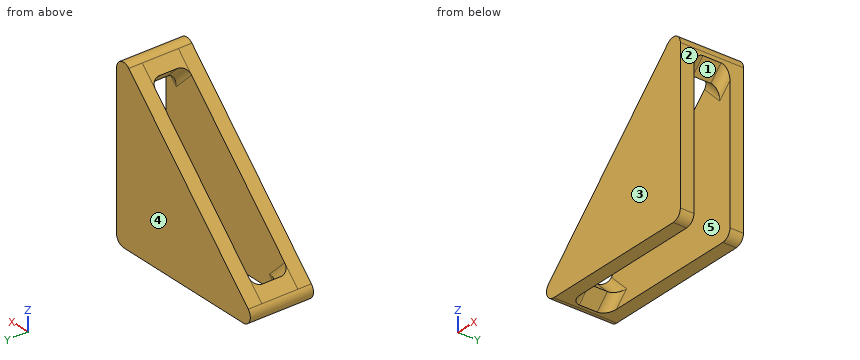
Autodesk Inventor part; units mm, degrees
ref_plane "YZ Plane" through (0, 0, 0) normal (1, 0, 0) x (0, 1, 0)
ref_plane "XZ Plane" through (0, 0, 0) normal (0, 1, 0) x (-1, 0, 0)
ref_plane "XY Plane" through (0, 0, 0) normal (0, 0, 1) x (1, 0, 0)
sketch "Sketch1" plane through (0, 0, 0) normal (0, 1, 0) x (-1, 0, 0)
  line L0 (0, 0) -> (-40, 0)
  line L1 (-40, 0) -> (-40, 40)
  line L2 (-40, 40) -> (0, 0)
  dimension "d0" = 40
  dimension "d1" = 40
  dimension "d2" = 56.5685
extrude "Extrusion1" add sketch "Sketch1" along normal blind 14
sketch "Sketch2" plane through (40, 0, 40) normal (-0.7071068, 0, 0.7071068) x (0.7071068, 0, 0.7071068)
  line L0 (-56.5685, 0) -> (-56.5685, 14) construction
  line L1 (-56.5685, 7) -> (0, 7) construction
  line L2 (0, 0) -> (0, 14) construction
  line L3 (-52.5685, 11) -> (-4, 11)
  line L4 (-4, 11) -> (-4, 3)
  line L5 (-4, 3) -> (-52.5685, 3)
  line L6 (-52.5685, 3) -> (-52.5685, 11)
  line L7 (-52.5685, 11) -> (-4, 3) construction
  line L8 (-4, 11) -> (-52.5685, 3) construction
  point P0 (-28.2843, 7)
  dimension "d5" = 4
  dimension "d6" = 4
  dimension "d20" = 8
extrude "Extrusion2" cut sketch "Sketch2" against normal blind 28.75
fillet "Fillet1" radius 2 4 edges at (40, 12.5, 0) (40, 1.5, 0) (40, 7, 40) (0, 7, 0)
sketch "Sketch4" plane through (5.6569, 3, 0) normal (0.7071068, 0, 0.7071068) x (0.7071068, 0, -0.7071068)
  line L0 (-3.8204, 0) -> (-3.8204, 8)
  line L1 (-3.8204, 0) -> (0, 0)
  line L2 (0, 8) -> (0, 0)
  line L3 (-3.8204, 8) -> (0, 8)
  point P0 (-4, -3)
extrude "Extrusion3" add sketch "Sketch4" along normal blind 4
sketch "Sketch5" plane through (40, 3, 34.3431) normal (-0.7071068, 0, -0.7071068) x (-0.7071068, 0, 0.7071068)
  line L0 (3.8204, 8) -> (3.8204, 0)
  line L1 (3.8204, 8) -> (0, 8)
  line L2 (0, 0) -> (0, 8)
  line L3 (3.8204, 0) -> (0, 0)
  point P0 (4, -3)
extrude "Extrusion4" add sketch "Sketch5" along normal blind 4
sketch "Sketch6" plane through (37.2986, 3, 37.0445) normal (-0.7071068, 0, 0.7071068) x (0.7071068, 0, 0.7071068)
  line L0 (0, 8) -> (0, 0)
  line L1 (-4, 8) -> (0, 8)
  line L2 (-4, 0) -> (-4, 8)
  line L3 (0, 0) -> (-4, 0)
  point P0 (-52.5685, -3)
extrude "Extrusion5" add sketch "Sketch6" along normal up to surface (0.1796 mm away)
sketch "Sketch7" plane through (2.9555, 3, 2.7014) normal (-0.7071068, 0, 0.7071068) x (0.7071068, 0, 0.7071068)
  line L0 (0, 0) -> (0, 8)
  line L1 (4, 0) -> (0, 0)
  line L2 (4, 8) -> (4, 0)
  line L3 (0, 8) -> (4, 8)
  point P0 (-4, -3)
extrude "Extrusion6" add sketch "Sketch7" along normal up to surface (0.1796 mm away)
fillet "Fillet2" radius 2 2 edges at (37.1716, 7, 37.1716) (2.8284, 7, 2.8284)
fillet "Fillet3" radius 2 8 edges at (7.0711, 11, 4.2426) (7.0711, 3, 4.2426) (35.7574, 3, 32.9289) (35.7574, 11, 32.9289) (7.0711, 11, 1.4142) (7.0711, 3, 1.4142) (38.5858, 3, 32.9289) (38.5858, 11, 32.9289)
properties part number "table-corners"
The listing builds one solid part. Answer for the finished solid, in the listing's coordinates (mm). Face numbers are marked on the shaded views. A direction names the side the tool comes from. Give positions to 0.01 mm unless a question says otherwise; leave off trailing zeros. Write each loop counter-clockwise with the first axis right and the second up, starting at its lowest first coordinate (ties: lowest second). Pieces come first, ordered by that corner, then holes. Notation, with made-up numbers: (61.5, -10) -> (110.5, -10) arc R38 cw to (110.5, 29) -> close; hole circle Ø2 at (-5.5, 85.5). An arc over 180 degrees is marked (long way). Use one line per item in the form item = value.
1) Section C-C on y = 6.75 is taken. Write down the section's boundary in (x, z), plus the area to 3 significant figures.
Result:
outline = (3.41, 3.41) arc R2 ccw to (4.83, 0) -> (5.66, 0) -> (8.49, 2.83) -> (5.66, 5.66) -> close; (34.34, 34.34) -> (37.17, 31.51) -> (40, 34.34) -> (40, 35.17) arc R2 ccw to (36.59, 36.59) -> close
area = 38.1 mm²
2) Straight lines are drawn through the part: probe 1 along Y at (x, z) = (14, 10); probe 2 along Z at (x, y) = (36.5, 5.75); probe 3 along Z at (x, y) = (6, 4). For each, find the intervals that lie inside material, in ascending order.
Result:
probe_1 = 0 to 3, 11 to 14
probe_2 = 32.19 to 36.5
probe_3 = 0 to 5.69
3) Section B-B on z = 25.5 is taken. Write down the section's boundary in (x, y), plus the area to 3 significant figures.
Result:
outline = (25.5, 0) -> (40, 0) -> (40, 3) -> (25.5, 3) -> close; (25.5, 11) -> (40, 11) -> (40, 14) -> (25.5, 14) -> close
area = 87.0 mm²
4) A tool of negligible diameter and unlimited length cuts with its end or side. For the marked faces 1 and 2, from which of +Z, -Z, +X, -X, +Y, -Y can it reach the whole face along a straight path? Write none if from no direction.
Result:
face_1 = -Z, +X
face_2 = +Z, -Z, +X, +Y, -Y
5) Section D-D on y = 1 is taken. Write down the section's boundary in (x, z).
Result:
outline = (3.41, 3.41) arc R2 ccw to (4.83, 0) -> (38, 0) arc R2 ccw to (40, 2) -> (40, 35.17) arc R2 ccw to (36.59, 36.59) -> close
6) Each of these flat-tipped pins is pushed along its axis until it touches: P1, Ø2, axis at x = 15, z = 16.5, coming from the -Y side; P2, Ø6, axis at y = 7, z = 30, coming from the +X side. Where does it stop, or does it pass through?
Result:
P1 = through
P2 = 38.66
7) Section A-A on x = 21 is taken. Write down the section's boundary in (y, z).
Result:
outline = (0, 0) -> (3, 0) -> (3, 21) -> (0, 21) -> close; (11, 0) -> (14, 0) -> (14, 21) -> (11, 21) -> close
8) For a pull along Y with two mould halves and no side action, classify the marked faces 3, 4 and 5 as +Y half, -Y half, draft (parallel to the pull), parting line (faces both ways), or undercut.
Result:
face_3 = -Y half
face_4 = +Y half
face_5 = undercut
